The listing builds one solid part. Answer for the finished solid, in the listing's coordinates (mm). A direction names the side the tool comes from. Coordinates: 2 decimals unless noted, no trailing zeros. Order: outer loops, then holes, each group sorted by start corner. A loop starts at its lowest first (then second) coordinate and runs counter-clockwise, first axis right, second up. Notation, with made-up numbers: (31, 78.25) -> (42, 78.25) arc R13 ccw to (42, 101.25) -> close; hole circle Ø5 at (16, 85.5). An arc over 180 degrees is marked (long way). Return JSON: item names as keys, results as strings.
```python
from build123d import *

# Parameters (mm, degrees)
EXTRUDE_1_DEPTH     = 2
SKETCH_2_R          = 0.8
CUT_EXTRUDE_1_DEPTH = 4
SKETCH_3_R          = 0.8
CUT_EXTRUDE_2_DEPTH = 4
SKETCH_4_R          = 0.8
CUT_EXTRUDE_3_DEPTH = 4
SKETCH_5_R          = 0.8
CUT_EXTRUDE_4_DEPTH = 4
SKETCH_9_R          = 1.5
EXTRUDE_2_DEPTH     = 1.5
SKETCH_10_R         = 0.8
EXTRUDE_3_DEPTH     = 40
SKETCH_11_R         = 0.8
EXTRUDE_4_DEPTH     = 40
SKETCH_15_W         = 2
SKETCH_15_H         = 34.731142246
SKETCH_15_W_2       = 34.731142246
SKETCH_15_H_2       = 2
EXTRUDE_6_DEPTH     = 1


with BuildPart() as part:
    # 草图1 → 凸台-拉伸1 (new body)
    with BuildSketch(Plane(origin=(0, 0, 0), x_dir=(1, 0, 0), z_dir=(0, 1, 0))):
        Polygon((3, -3), (6, -3), (10, -1), (10, 1), (6, 3), (3, 3), (3, 6), (1, 10), (-1, 10), (-3, 6), (-3, 3), (-6, 3), (-10, 1), (-10, -1), (-6, -3), (-3, -3), (-3, -6), (-1, -10), (1, -10), (3, -6), align=None)
    extrude(amount=EXTRUDE_1_DEPTH)

    # 草图2 → 切除-拉伸1 (cut)
    with BuildSketch(Plane.XY.offset(10)):
        with Locations((0, 1)):
            Circle(SKETCH_2_R)
    extrude(amount=-CUT_EXTRUDE_1_DEPTH, mode=Mode.SUBTRACT)

    # 草图3 → 切除-拉伸2 (cut)
    with BuildSketch(Plane(origin=(10, 0, 0), x_dir=(0, 0, -1), z_dir=(1, 0, 0))):
        with Locations((0, 1)):
            Circle(SKETCH_3_R)
    extrude(amount=-CUT_EXTRUDE_2_DEPTH, mode=Mode.SUBTRACT)

    # 草图4 → 切除-拉伸3 (cut)
    with BuildSketch(Plane(origin=(0, 0, -10), x_dir=(-1, 0, 0), z_dir=(0, 0, -1))):
        with Locations((0, 1)):
            Circle(SKETCH_4_R)
    extrude(amount=-CUT_EXTRUDE_3_DEPTH, mode=Mode.SUBTRACT)

    # 草图5 → 切除-拉伸4 (cut)
    with BuildSketch(Plane.ZY.offset(10)):
        with Locations((0, 1)):
            Circle(SKETCH_5_R)
    extrude(amount=-CUT_EXTRUDE_4_DEPTH, mode=Mode.SUBTRACT)

    # 草图9 → 凸台-拉伸2 (add)
    with BuildSketch(Plane(origin=(-1.202081528, 0, 1.202081528), x_dir=(0.707106781, 0, 0.707106781), z_dir=(-0.707106781, 0, 0.707106781))):
        with BuildLine():
            Line((2.5, 5.5), (2.5, 4))
            Line((2.5, 4), (4, 4))
            Line((4, 4), (4, 2))
            Line((4, 2), (-4, 2))
            Line((-4, 2), (-4, 4))
            Line((-4, 4), (-2.5, 4))
            Line((-2.5, 4), (-2.5, 5.5))
            ThreePointArc((-2.5, 5.5), (0, 8), (2.5, 5.5))
        make_face()
        with Locations((0, 5.5)):
            Circle(SKETCH_9_R, mode=Mode.SUBTRACT)
    extrude_2 = extrude(amount=EXTRUDE_2_DEPTH)

    # 镜向1: 凸台-拉伸2 across plane
    add(extrude_2.mirror(Plane(origin=(0, 0, 0), x_dir=(0.707106781, 0, 0.707106781), z_dir=(-0.707106781, 0, 0.707106781))))

    # 草图10 → 凸台-拉伸3 (add)
    with BuildSketch(Plane.ZY.offset(6)):
        with Locations((0, 1)):
            Circle(SKETCH_10_R)
    extrude_3 = extrude(amount=EXTRUDE_3_DEPTH)

    # 草图11 → 凸台-拉伸4 (add)
    with BuildSketch(Plane.XY.offset(6)):
        with Locations((0, 1)):
            Circle(SKETCH_11_R)
    extrude_4 = extrude(amount=EXTRUDE_4_DEPTH)

    # 镜向2: 凸台-拉伸4 across plane
    add(extrude_4.mirror(Plane.XY))

    # 镜向3: 凸台-拉伸3 across plane
    add(extrude_3.mirror(Plane(origin=(0, 0, 0), x_dir=(0, 0, 1), z_dir=(1, 0, 0))))

    # 草图12 → 旋转1 (revolve)
    with BuildSketch(Plane(origin=(0, 0, 0), x_dir=(0, 0, -1), z_dir=(1, 0, 0))):
        with BuildLine():
            Line((-47.5, 1), (-44.5, 1))
            ThreePointArc((-44.5, 1), (-46, 2.5), (-47.5, 1))
        make_face()
    revolve_1 = revolve(axis=Axis((0, 1, 47.5), (0, 0, -1)))

    # 草图14 → 旋转2 (revolve)
    with BuildSketch(Plane.XY):
        with BuildLine():
            Line((-47.5, 1), (-44.5, 1))
            ThreePointArc((-44.5, 1), (-46, 2.5), (-47.5, 1))
        make_face()
    revolve_2 = revolve(axis=Axis((-47.5, 1, 0), (1, 0, 0)))

    # 镜向4: 旋转1 across plane
    add(revolve_1.mirror(Plane.XY))

    # 镜向5: 旋转2 across plane
    add(revolve_2.mirror(Plane(origin=(0, 0, 0), x_dir=(0, 0, 1), z_dir=(1, 0, 0))))

    # 草图15 → 凸台-拉伸6 (add)
    with BuildSketch(Plane(origin=(0, 0, 0), x_dir=(1, 0, 0), z_dir=(0, 1, 0))):
        with Locations((0, 27.365571123)):
            Rectangle(SKETCH_15_W, SKETCH_15_H)
        with Locations((27.365571123, 0)):
            Rectangle(SKETCH_15_W_2, SKETCH_15_H_2)
        with Locations((0, -27.365571123)):
            Rectangle(SKETCH_15_W, SKETCH_15_H)
        with Locations((-27.365571123, 0)):
            Rectangle(SKETCH_15_W_2, SKETCH_15_H_2)
    extrude(amount=EXTRUDE_6_DEPTH)


solid = part.part
```
Item 1: Flat-ended cylindrical pins translate along their axes: pin 1 (1.1 mm diameter, centred on x = 0.5, y = 0.5, fed in from -Z); pin 2 (0.5 mm diameter, centred on y = 0.5, z = 19, fed in from +X); pin 3 (0.5 mm diameter, centred on y = 0.5, z = 0.5, fed in from +X); pin 4 (4 mm diameter, centred on y = 4, z = 11, fed in from +X). Find the tip coordinate at first contact, or state that the pin passes through.
Answer list:
{"pin 1": "z = -47.49", "pin 2": "x = 1", "pin 3": "x = 47.43", "pin 4": "through"}
Item 2: Determine the mould class of faces 1 (the flat face through (-4, 4, -1)), 2 (the flat face through (0, 0, 0)), 3 (the cylindrical face through (-2, 8, 2)) for opening direction X: pulls with the +X half, pulls with the -X half, needs draft (parallel to the pull), parting line crosses it, or undercut.
Answer list:
{"face 1": "needs draft", "face 2": "undercut", "face 3": "parting line crosses it"}
Item 3: Which of the six approach directions +Z, -Z, +X, -X, +Y, -Y give full straight-line access (tool end or side, diameter ignored) to faces 4 (the flat face through (1, 4, 4)), 5 (the flat face through (-1.162, 3.709, 1.242)), 6 (the cylindrical face through (-1.955, 4.036, 1.495)), 7 (the flat face through (-1, 4, -4))?
Answer list:
{"face 4": "+Z, +X, +Y", "face 5": "+Y", "face 6": "none", "face 7": "-Z, -X, +Y"}
Item 4: The part is cut by section A-A on x = 33. Determine the outline of the cut face in (y, z).
Answer list:
{"outline": "(0, -1) -> (1, -1) -> (1, -0.8) arc R0.8 ccw to (1, 0.8) -> (1, 1) -> (0, 1) -> close"}
Item 5: The part is cut by section B-B on z = -11.5. Determine the outline of the cut face in (x, y).
Answer list:
{"outline": "(-1, 0) -> (1, 0) -> (1, 1) -> (0.8, 1) arc R0.8 ccw to (-0.8, 1) -> (-1, 1) -> close"}
Item 6: Find the intervals of material crossed by probe 1 along X at (y, z) = (0.75, 36); probe 2 along X at (y, z) = (1.5, -26), in increasing order.
Answer list:
{"probe 1": "-1 to 1", "probe 2": "-0.62 to 0.62"}
